from build123d import *

# Parameters (mm, degrees)
BASE_R                                               = 121
BASE_R_2                                             = 115
BASE_EXTRUDE_DEPTH                                   = 40
CSK_FOR_M5_COUNTERSUNK_RAISED_HEAD_SCREW_D           = 5.5
CSK_FOR_M5_COUNTERSUNK_RAISED_HEAD_SCREW_DEPTH       = 20
CSK_FOR_M5_COUNTERSUNK_RAISED_HEAD_SCREW_CSINK_D     = 10.4
CSK_FOR_M5_COUNTERSUNK_RAISED_HEAD_SCREW_CSINK_ANGLE = 90
CSK_FOR_M5_COUNTERSUNK_RAISED_HEAD_SCREW_TIP         = 1.652366702


with BuildPart() as part:
    # Base → Base-Extrude (new body)
    with BuildSketch(Plane(origin=(0, 0, 0), x_dir=(1, 0, 0), z_dir=(0, 1, 0))):
        with Locations(Location((0, 0, 0), (0, 0, 270))):
            Circle(BASE_R)
        with Locations(Location((0, 0, 0), (0, 0, 270))):
            Circle(BASE_R_2, mode=Mode.SUBTRACT)
    extrude(amount=BASE_EXTRUDE_DEPTH)

    # CSK for M5 Countersunk Raised Head Screw1
    with Locations(Plane(origin=(37.968714772, -4, -14.434938782), x_dir=(-1, 0, 0), z_dir=(0, -1, 0))):
        with Locations((-45.469885408, -97.873538962), (-80.031285228, -14.434938782), (-45.469885408, 69.003661398), (37.968714772, 103.565061218), (121.407314952, 69.003661398), (155.968714772, -14.434938782), (121.407314952, -97.873538962), (37.968714772, -132.434938782)):
            CounterSinkHole(CSK_FOR_M5_COUNTERSUNK_RAISED_HEAD_SCREW_D / 2, CSK_FOR_M5_COUNTERSUNK_RAISED_HEAD_SCREW_CSINK_D / 2, depth=CSK_FOR_M5_COUNTERSUNK_RAISED_HEAD_SCREW_DEPTH, counter_sink_angle=CSK_FOR_M5_COUNTERSUNK_RAISED_HEAD_SCREW_CSINK_ANGLE)
            with Locations((0, 0, -(CSK_FOR_M5_COUNTERSUNK_RAISED_HEAD_SCREW_DEPTH + CSK_FOR_M5_COUNTERSUNK_RAISED_HEAD_SCREW_TIP / 2))):  # 118° drill point
                Cone(0, CSK_FOR_M5_COUNTERSUNK_RAISED_HEAD_SCREW_D / 2, CSK_FOR_M5_COUNTERSUNK_RAISED_HEAD_SCREW_TIP, mode=Mode.SUBTRACT)


solid = part.part
The listing builds one solid part. Answer for the finished solid, in the listing's coordinates (mm). A direction names the side the tool comes from. Coordinates: 2 decimals unless noted, no trailing zeros. Order: outer loops, then holes, each group sorted by start corner. A loop starts at its lowest first (then second) coordinate and runs counter-clockwise, first axis right, second up. Notation, with made-up numbers: M -23,63.5 L 9,63.5 A21 cw 9,72.5 Z; hole C 9,40 d4. An arc over 180 degrees is marked long. Use CSV: the item, a comma, the result in double quotes.
Q1. Section D-D (y = 37) is taken. Determine the outline of the cut face in (x, z), then the cut area to 3 significant figures.
Here are the results:
outline,"C 0,0 d242; hole C 0,0 d230"
area,"4,450 mm2"
Q2. A tool of negligible diameter and unlimited length cuts with its end or side. For faces 1 (the cylindrical face through (-112.265, 19.72, -24.93)), 2 (the cylindrical face through (-0.596, 8.112, 120.685)), from which of +Z, -Z, +X, -X, +Y, -Y can it reach the whole face along a straight path? Write none if from no direction.
Here are the results:
face 1,"+Y, -Y"
face 2,"-Y"
Q3. Section C-C (y = 13) is taken. Give the number of separate pieces and of enclosed holes in the cut face, then the cut area to 3 significant figures.
Here are the results:
separate pieces,"1"
enclosed holes,"9"
area,"4,260 mm2"
Q4. Straight lines are drawn through the part: L1, parallel to X at y = 10, z = 1; L2, parallel to Z at x = 84.5, y = 4.5; L3, parallel to X at y = 21, z = 83. For each, find the intervals that lie inside material, in ascending order.
Here are the results:
L1,"-121 to -120.56, -115.44 to -115, 115 to 115.44, 120.56 to 121"
L2,"-86.61 to -85.98, -80.9 to -78, 78 to 80.9, 85.98 to 86.61"
L3,"-88.05 to -79.6, 79.6 to 88.05"
Q5. Given pin 1 Ø6 at (x, y) = (96.5, 27) entering from +Z; pin 2 Ø4 at (y, z) = (8, 41) entering from -X; pin 3 Ø4 at (y, z) = (30, -24.5) entering from +X, each flat-ended and moving along its own axis, determine where each tip first touches the part or whether it passes through.
Here are the results:
pin 1,"z = 76.8"
pin 2,"x = -114.54"
pin 3,"x = 118.89"
Q6. Determine the mould class of faces 3 (the cylindrical face through (-118.123, 19.72, -26.23)), 4 (the flat face through (-44, 40, 107)), 5 (the conical face through (-117.523, 17.365, -0.021)) for opening direction X: pulls with the +X half, pulls with the -X half, needs draft (parallel to the pull), parting line crosses it, or undercut.
Here are the results:
face 3,"parting line crosses it"
face 4,"needs draft"
face 5,"undercut"
Q7. Section B-B (x = -100) is taken. Determine the outline of the cut face in (y, z), then the cut area to 3 significant figures.
Here are the results:
outline,"M 0,-68.12 L 40,-68.12 L 40,-56.79 L 0,-56.79 Z; M 0,56.79 L 40,56.79 L 40,68.12 L 0,68.12 Z"
area,"907 mm2"
Q8. Section A-A (z = -92) is taken. Determine the outline of the cut face in (x, y).
Here are the results:
outline,"M -78.59,0 L -69,0 L -69,40 L -78.59,40 Z; M 69,0 L 78.59,0 L 78.59,40 L 69,40 Z"
